```python
from build123d import *

# Parameters (mm, degrees)
EXTRUDE_1_DEPTH          = 80
SKETCH_3_R               = 37.25
CUT_EXTRUDE_1_DEPTH      = 10.3
SKETCH_4_R               = 22.7
CUT_EXTRUDE_2_DEPTH      = 65
CUT_EXTRUDE_3_DEPTH      = 138.477270849
SKETCH_6_W               = 160
SKETCH_6_H               = 12
EXTRUDE_2_DEPTH          = 80
SKETCH_8_R               = 5.5
CUT_EXTRUDE_4_DEPTH      = 6.8
SKETCH_9_R               = 3.3
CUT_EXTRUDE_5_DEPTH      = 179.44887223
RIB_START                = -5
RIB_1_DEPTH              = 10
PATTERN_CIRCULAR_1_COUNT = 4
EXTRUDE_3_DEPTH          = 0.1
EXTRUDE_4_DEPTH          = 0.2


# Read off the part's stored shape, not the designer's step: 筋1, 高级异型孔1, 高级异型孔2
with BuildPart() as part:
    # 草图1 → 凸台-拉伸1 (new body)
    with BuildSketch(Plane(origin=(0, 0, 0), x_dir=(1, 0, 0), z_dir=(0, 1, 0))):
        with BuildLine():
            Line((-50, -100), (0, -100))
            Line((0, -100), (0, -37.3))
            ThreePointArc((0, -37.3), (-37.3, 0), (0, 37.3))
            Line((0, 37.3), (0, 60))
            Line((0, 60), (-50, 60))
            Line((-50, 60), (-50, -100))
        make_face()
        with BuildLine():
            Line((0, -37.3), (0, -100))
            Line((0, -100), (50, -100))
            Line((50, -100), (50, 60))
            Line((50, 60), (0, 60))
            Line((0, 60), (0, 37.3))
            ThreePointArc((0, 37.3), (26.375082938, 26.375082938), (37.3, 0))
            ThreePointArc((37.3, 0), (26.375082938, -26.375082938), (0, -37.3))
        make_face()
        with BuildLine():
            ThreePointArc((0, 37.3), (-37.3, 0), (0, -37.3))
            Line((0, -37.3), (0, -16))
            ThreePointArc((0, -16), (-16, 0), (0, 16))
            Line((0, 16), (0, 37.3))
        make_face()
        with BuildLine():
            Line((0, -16), (0, -37.3))
            ThreePointArc((0, -37.3), (26.375082938, -26.375082938), (37.3, 0))
            ThreePointArc((37.3, 0), (26.375082938, 26.375082938), (0, 37.3))
            Line((0, 37.3), (0, 16))
            ThreePointArc((0, 16), (11.313708499, 11.313708499), (16, 0))
            ThreePointArc((16, 0), (11.313708499, -11.313708499), (0, -16))
        make_face()
    extrude(amount=EXTRUDE_1_DEPTH)

    # 草图3 → 切除-拉伸1 (cut)
    with BuildSketch(Plane(origin=(0, 80, 0), x_dir=(1, 0, 0), z_dir=(0, 1, 0))):
        with Locations(Location((0, 0, 0), (0, 0, 270))):
            Circle(SKETCH_3_R)
    extrude(amount=-CUT_EXTRUDE_1_DEPTH, mode=Mode.SUBTRACT)

    # 草图4 → 切除-拉伸2 (cut)
    with BuildSketch(Plane(origin=(0, 80, 0), x_dir=(1, 0, 0), z_dir=(0, 1, 0))):
        with Locations(Location((0, 0, 0), (0, 0, 270))):
            Circle(SKETCH_4_R)
    extrude(amount=-CUT_EXTRUDE_2_DEPTH, mode=Mode.SUBTRACT)

    # 草图5 → 切除-拉伸3 (cut, through all)
    with BuildSketch(Plane(origin=(0, 80, 0), x_dir=(1, 0, 0), z_dir=(0, 1, 0))):
        with BuildLine():
            ThreePointArc((-50, 1.43e-07), (7.1e-08, 50), (50, 0))
            Line((50, 0), (50, 60))
            Line((50, 60), (-50, 60))
            Line((-50, 60), (-50, 1.43e-07))
        make_face()
    extrude(amount=-CUT_EXTRUDE_3_DEPTH, mode=Mode.SUBTRACT)

    # 草图6 → 凸台-拉伸2 (add)
    with BuildSketch(Plane(origin=(0, 80, 0), x_dir=(1, 0, 0), z_dir=(0, 1, 0))):
        with Locations((0, -94)):
            Rectangle(SKETCH_6_W, SKETCH_6_H)
    extrude(amount=-EXTRUDE_2_DEPTH)

    # 草图8 → 切除-拉伸4 (cut)
    with BuildSketch(Plane(origin=(0, 0, 88), x_dir=(-1, 0, 0), z_dir=(0, 0, -1))):
        with Locations((63.5, 65.4)):
            Circle(SKETCH_8_R)
        with Locations(Location((63.5, 14.6, 0), (0, 0, 180))):
            Circle(SKETCH_8_R)
    cut_extrude_4 = extrude(amount=-CUT_EXTRUDE_4_DEPTH, mode=Mode.SUBTRACT)

    # 草图9 → 切除-拉伸5 (cut, through all)
    with BuildSketch(Plane(origin=(0, 0, 88), x_dir=(-1, 0, 0), z_dir=(0, 0, -1))):
        with Locations((63.5, 65.4)):
            Circle(SKETCH_9_R)
        with Locations((63.5, 14.6)):
            Circle(SKETCH_9_R)
    cut_extrude_5 = extrude(amount=-CUT_EXTRUDE_5_DEPTH, mode=Mode.SUBTRACT)

    # 镜向1: 切除-拉伸4, 切除-拉伸5 across plane
    add(cut_extrude_4.mirror(Plane(origin=(0, 0, 0), x_dir=(0, 0, 1), z_dir=(1, 0, 0))), mode=Mode.SUBTRACT)
    add(cut_extrude_5.mirror(Plane(origin=(0, 0, 0), x_dir=(0, 0, 1), z_dir=(1, 0, 0))), mode=Mode.SUBTRACT)

    # 筋1 outline → 筋1 (add)
    with BuildSketch(Plane(origin=(0, 40, 0), x_dir=(1, 0, 0), z_dir=(0, 1, 0)).offset(RIB_START)):
        Polygon((-50, -58), (-80, -88), (-50, -88), align=None)
    rib_1 = extrude(amount=RIB_1_DEPTH)

    # 镜向2: 筋1 across plane
    add(rib_1.mirror(Plane(origin=(0, 0, 0), x_dir=(0, 0, 1), z_dir=(1, 0, 0))))

    # 高级异型孔1 outline → 高级异型孔1 (revolve, cut)
    with BuildSketch(Plane(origin=(21.213203436, 0, -21.213203436), x_dir=(1, 0, 0), z_dir=(0, 0, 1))):
        Polygon((2.3, 68.5), (3.6, 68.5), (3.6, 69.7), (0, 69.7), (0, 57.11802058), (2.3, 58.5), align=None)
    other_1 = revolve(axis=Axis((21.213203436, 0, -21.213203436), (0, 1, 0)), mode=Mode.SUBTRACT)

    # 阵列(圆周)1: 高级异型孔1 ×4 about axis
    pattern_circular_1_axis = Axis((0, 0, 0), (0, 1, 0))
    for i in range(1, PATTERN_CIRCULAR_1_COUNT):
        add(other_1.rotate(pattern_circular_1_axis, i * 360 / PATTERN_CIRCULAR_1_COUNT), mode=Mode.SUBTRACT)

    # 高级异型孔2 outline → 高级异型孔2 (revolve, cut)
    with BuildSketch(Plane(origin=(15, 0, 55), x_dir=(1, 0, 0), z_dir=(0, 0, 1))):
        Polygon((3.6, 0), (3.6, 1.5), (2.3, 1.5), (2.3, 11.5), (0, 12.88197942), (0, 0), align=None)
    revolve(axis=Axis((15, 0, 55), (0, 1, 0)), mode=Mode.SUBTRACT)

    # Other 2 2 outline → Other 2 2 (revolve, cut)
    with BuildSketch(Plane(origin=(-15, 0, 55), x_dir=(1, 0, 0), z_dir=(0, 0, 1))):
        Polygon((0, 0), (3.6, 0), (3.6, 1.5), (2.3, 1.5), (2.3, 11.5), (0, 12.88197942), align=None)
    revolve(axis=Axis((-15, 0, 55), (0, 1, 0)), mode=Mode.SUBTRACT)

    # 草图14 → 凸台-拉伸3 (add)
    with BuildSketch(Plane.XZ.offset(-1.5)):
        with BuildLine():
            Line((-16.327905619, 57.3), (-15.607120186, 58.548436991))
            ThreePointArc((-15.607120186, 58.548436991), (-16.8, 58.117691454), (-17.769476485, 57.3))
            Line((-17.769476485, 57.3), (-16.327905619, 57.3))
        make_face()
        with BuildLine():
            Line((-17.655811238, 55), (-16.327905619, 57.3))
            Line((-16.327905619, 57.3), (-17.769476485, 57.3))
            ThreePointArc((-17.769476485, 57.3), (-18.117691454, 56.8), (-18.376596671, 56.248436991))
            Line((-18.376596671, 56.248436991), (-17.655811238, 55))
        make_face()
        with BuildLine():
            Line((-18.376596671, 53.751563009), (-17.655811238, 55))
            Line((-17.655811238, 55), (-18.376596671, 56.248436991))
            ThreePointArc((-18.376596671, 56.248436991), (-18.6, 55), (-18.376596671, 53.751563009))
        make_face()
        with BuildLine():
            Line((-15.607120186, 51.451563009), (-16.327905619, 52.7))
            Line((-16.327905619, 52.7), (-17.769476485, 52.7))
            ThreePointArc((-17.769476485, 52.7), (-16.8, 51.882308546), (-15.607120186, 51.451563009))
        make_face()
        with BuildLine():
            Line((-13.672094381, 52.7), (-16.327905619, 52.7))
            Line((-16.327905619, 52.7), (-15.607120186, 51.451563009))
            ThreePointArc((-15.607120186, 51.451563009), (-15, 51.4), (-14.392879814, 51.451563009))
            Line((-14.392879814, 51.451563009), (-13.672094381, 52.7))
        make_face()
        with BuildLine():
            Line((-12.230523515, 52.7), (-13.672094381, 52.7))
            Line((-13.672094381, 52.7), (-14.392879814, 51.451563009))
            ThreePointArc((-14.392879814, 51.451563009), (-13.2, 51.882308546), (-12.230523515, 52.7))
        make_face()
        with BuildLine():
            Line((-11.623403329, 56.248436991), (-12.344188762, 55))
            Line((-12.344188762, 55), (-11.623403329, 53.751563009))
            ThreePointArc((-11.623403329, 53.751563009), (-11.456290925, 54.365865951), (-11.4, 55))
            ThreePointArc((-11.4, 55), (-11.456290925, 55.634134049), (-11.623403329, 56.248436991))
        make_face()
        with BuildLine():
            Line((-12.230523515, 57.3), (-13.672094381, 57.3))
            Line((-13.672094381, 57.3), (-12.344188762, 55))
            Line((-12.344188762, 55), (-11.623403329, 56.248436991))
            ThreePointArc((-11.623403329, 56.248436991), (-11.882308546, 56.8), (-12.230523515, 57.3))
        make_face()
        with BuildLine():
            ThreePointArc((-12.230523515, 57.3), (-13.2, 58.117691454), (-14.392879814, 58.548436991))
            Line((-14.392879814, 58.548436991), (-13.672094381, 57.3))
            Line((-13.672094381, 57.3), (-12.230523515, 57.3))
        make_face()
    extrude_3 = extrude(amount=EXTRUDE_3_DEPTH)

    # 草图14<3> → 凸台-拉伸4 (add)
    with BuildSketch(Plane.XZ.offset(-1.5)):
        with BuildLine():
            Line((-16.327905619, 52.7), (-17.655811238, 55))
            Line((-17.655811238, 55), (-18.376596671, 53.751563009))
            ThreePointArc((-18.376596671, 53.751563009), (-18.117691454, 53.2), (-17.769476485, 52.7))
            Line((-17.769476485, 52.7), (-16.327905619, 52.7))
        make_face()
        with BuildLine():
            Line((-18.376596671, 53.751563009), (-17.655811238, 55))
            Line((-17.655811238, 55), (-18.376596671, 56.248436991))
            ThreePointArc((-18.376596671, 56.248436991), (-18.6, 55), (-18.376596671, 53.751563009))
        make_face()
        with BuildLine():
            Line((-15.607120186, 51.451563009), (-16.327905619, 52.7))
            Line((-16.327905619, 52.7), (-17.769476485, 52.7))
            ThreePointArc((-17.769476485, 52.7), (-16.8, 51.882308546), (-15.607120186, 51.451563009))
        make_face()
        with BuildLine():
            Line((-12.230523515, 52.7), (-13.672094381, 52.7))
            Line((-13.672094381, 52.7), (-14.392879814, 51.451563009))
            ThreePointArc((-14.392879814, 51.451563009), (-13.2, 51.882308546), (-12.230523515, 52.7))
        make_face()
        with BuildLine():
            Line((-11.623403329, 53.751563009), (-12.344188762, 55))
            Line((-12.344188762, 55), (-13.672094381, 52.7))
            Line((-13.672094381, 52.7), (-12.230523515, 52.7))
            ThreePointArc((-12.230523515, 52.7), (-11.882308546, 53.2), (-11.623403329, 53.751563009))
        make_face()
        with BuildLine():
            Line((-11.623403329, 56.248436991), (-12.344188762, 55))
            Line((-12.344188762, 55), (-11.623403329, 53.751563009))
            ThreePointArc((-11.623403329, 53.751563009), (-11.456290925, 54.365865951), (-11.4, 55))
            ThreePointArc((-11.4, 55), (-11.456290925, 55.634134049), (-11.623403329, 56.248436991))
        make_face()
        with BuildLine():
            ThreePointArc((-12.230523515, 57.3), (-13.2, 58.117691454), (-14.392879814, 58.548436991))
            Line((-14.392879814, 58.548436991), (-13.672094381, 57.3))
            Line((-13.672094381, 57.3), (-12.230523515, 57.3))
        make_face()
        with BuildLine():
            ThreePointArc((-14.392879814, 58.548436991), (-15, 58.6), (-15.607120186, 58.548436991))
            Line((-15.607120186, 58.548436991), (-16.327905619, 57.3))
            Line((-16.327905619, 57.3), (-13.672094381, 57.3))
            Line((-13.672094381, 57.3), (-14.392879814, 58.548436991))
        make_face()
        with BuildLine():
            Line((-16.327905619, 57.3), (-15.607120186, 58.548436991))
            ThreePointArc((-15.607120186, 58.548436991), (-16.8, 58.117691454), (-17.769476485, 57.3))
            Line((-17.769476485, 57.3), (-16.327905619, 57.3))
        make_face()
    extrude_4 = extrude(amount=EXTRUDE_4_DEPTH)

    # 镜向3: 凸台-拉伸3, 凸台-拉伸4 across plane
    add(extrude_3.mirror(Plane(origin=(0, 0, 0), x_dir=(0, 0, 1), z_dir=(1, 0, 0))))
    add(extrude_4.mirror(Plane(origin=(0, 0, 0), x_dir=(0, 0, 1), z_dir=(1, 0, 0))))


solid = part.part
```
Can you work these out from the model? Positions are in its coordinate system, mm. A direction names the side the tool comes from. Give positions to 0.01 mm unless a question says otherwise; leave off trailing zeros. Loops run counter-clockwise (first coordinate to the right, second up) from the corner with the lowest first, then second, coordinate; pieces in that order, holes last. Notation, with made-up numbers: M -15,3.5 L 28,3.5 A20 cw 28,8.5 Z; hole C 46.5,17.25 d10. An arc over 180 degrees is marked long. Answer in a Markdown table with one row per item.
1. If I drill on line 1 along Y through (x, z) = (-63, 90); line 2 along Y through (x, z) = (-63.5, 96.95); line 3 along X through (y, z) = (51.5, 0), over which ranges is the centre line in solid material (lowest first)?
Taken from the geometry:
| item | result |
|---|---|
| line 1 | y = 0 to 9.12, 20.08 to 59.92, 70.88 to 80 |
| line 2 | y = 0 to 11.3, 17.9 to 62.1, 68.7 to 80 |
| line 3 | x = -50 to -22.7, 22.7 to 50 |
2. Suppose I cut it at B-B on y = 47. Write out the boundary of the cut face in (x, z), plus the area to 3 significant figures.
Taken from the geometry:
| item | result |
|---|---|
| outline | M -80,88 L -50,88 L -50,0 A50 ccw 50,0 L 50,88 L 80,88 L 80,100 L -80,100 Z; hole C 0,0 d45.4 |
| area | 13,000 mm² |
3. Thinking about a two-plate mould opening in Z: for faces 1 (the cylindrical face through (-23.494, 63.57, -20.914)), 2 (the cylindrical face through (61.07, 67.63, 97.36)), 3 (the flat face through (-61, 17, 94.8)), which applies, released by +Z, released by -Z, zero draft, split by the parting line, or undercut?
Taken from the geometry:
| item | result |
|---|---|
| face 1 | undercut |
| face 2 | zero draft |
| face 3 | released by -Z |
4. Which directions (+Z, -Z, +X, -X, +Y, -Y) give clear straight access to the entire face, cutting with the end or side of a thin tool? Please do faces 4 (the cylindrical face through (20.914, 63.57, -23.494)), 5 (the flat face through (65, 22, 88)), 6 (the cylindrical face through (-68.995, 14.358, 91.352)), 7 (the flat face through (-69, 18, 88)), 8 (the flat face through (50, 39, 45)).
Taken from the geometry:
| item | result |
|---|---|
| face 4 | +Y |
| face 5 | -Z, +X, -Y |
| face 6 | -Z |
| face 7 | -Z, -X, -Y |
| face 8 | -Z, +X |
5. Suppose I cut it at A-A on x = -63.5. Write out the boundary of the cut face in (y, z), plus the area to 3 significant figures.
Taken from the geometry:
| item | result |
|---|---|
| outline | M 0,88 L 9.1,88 L 9.1,94.8 L 11.3,94.8 L 11.3,100 L 0,100 Z; M 17.9,94.8 L 20.1,94.8 L 20.1,88 L 35,88 L 35,71.5 L 45,71.5 L 45,88 L 59.9,88 L 59.9,94.8 L 62.1,94.8 L 62.1,100 L 17.9,100 Z; M 68.7,94.8 L 70.9,94.8 L 70.9,88 L 80,88 L 80,100 L 68.7,100 Z |
| area | 907 mm² |
6. For pin 1 Ø1.3 at (x, z) = (-13.5, 53.5) entering from -Y; pin 2 Ø12.5 at (x, y) = (63.5, 14.6) entering from -Z; pin 3 Ø3 at (x, z) = (-3.5, 17.5) entering from -Y; pin 4 Ø8.5 at (x, z) = (-21.21, -21.21) entering from +Y, each with a flat end and sliding along its axis, tell me the tip position at first contact or that it passes through.
Taken from the geometry:
| item | result |
|---|---|
| pin 1 | stops at y = 1.3 |
| pin 2 | stops at z = 88 |
| pin 3 | stops at y = 0 |
| pin 4 | stops at y = 69.7 |
7. Suppose I cut it at C-C on z = 9.5. Write out the boundary of the cut face in (x, y).
Taken from the geometry:
| item | result |
|---|---|
| outline | M -50,0 L -12.87,0 L -12.87,15 L -20.62,15 L -20.62,69.7 L -36.02,69.7 L -36.02,80 L -50,80 Z; M 12.87,0 L 50,0 L 50,80 L 36.02,80 L 36.02,69.7 L 20.62,69.7 L 20.62,15 L 12.87,15 Z |
